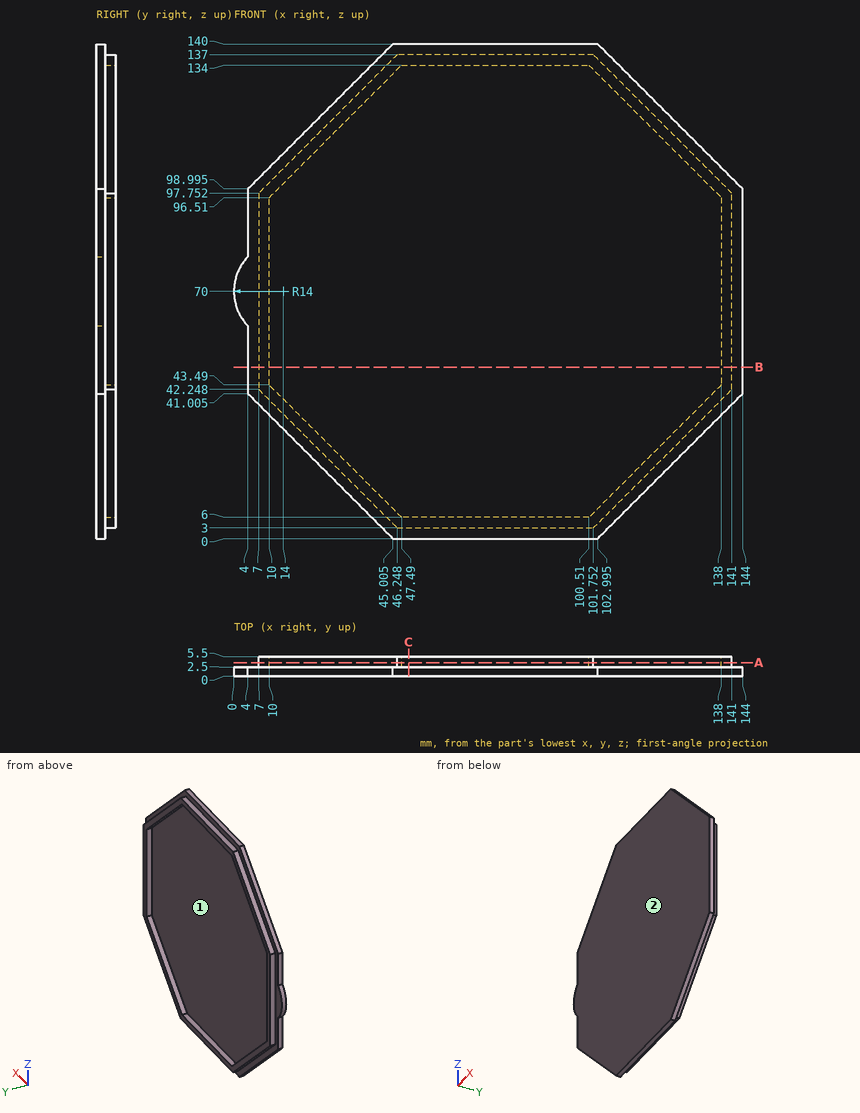
Can you work these out from the drawing? Everything is in mm from the part's minimum corner. Round coordinates to 2 decimals unless told otherwise and drop trailing zeros. Loops run counter-clockwise (first coordinate to the right, second up) from the corner with the lowest first, then second, coordinate; pieces in that order, holes last.
1. If we section it at A-A on y = 3.75: Write out the boundary of the cut face in (x, z), plus the area to 3 significant figures.
Answer list:
outline: (7, 42.25) - (46.25, 3) - (101.75, 3) - (141, 42.25) - (141, 97.75) - (101.75, 137) - (46.25, 137) - (7, 97.75) - close; hole (10, 43.49) - (47.49, 6) - (100.51, 6) - (138, 43.49) - (138, 96.51) - (100.51, 134) - (47.49, 134) - (10, 96.51) - close
area: 1,300 mm2
2. We'd pull the mould along Z, two halves only. Please class the marked faces 1 and 2: +Z half, -Z half, draft (parallel to the pull), parting line (faces both ways), or undercut.
Answer list:
face 1: undercut
face 2: draft
3. For P1, Ø3, axis at x = 79, y = 1.5, coming from the -Z side; P2, Ø2.5, axis at x = 73.5, y = 4, coming from the -Z side; P3, Ø2.5, axis at y = 4, z = 80, coming from the +X side; P4, Ø3, axis at y = 1, z = 92, coming from the -X side, each with a flat end and sliding along its axis, tell me the tip position at first contact or that it passes through.
Answer list:
P1: stops at z = 0
P2: stops at z = 3
P3: stops at x = 141
P4: stops at x = 4
4. If I drill on line 1 along X through (y, z) = (4.3, 64.5); line 2 along Y through (x, z) = (83.5, 60.5); line 3 along Z through (x, y) = (43.5, 2.7), over which ranges is the centre line in solid material (lowest first)?
Answer list:
line 1: x = 7 to 10, 138 to 141
line 2: y = 0 to 2.5
line 3: z = 5.75 to 9.99, 130.01 to 134.25
5. If we section it at C-C on x = 49.5: Write out the boundary of the cut face in (y, z).
Answer list:
outline: (0, 0) - (2.5, 0) - (2.5, 3) - (5.5, 3) - (5.5, 6) - (2.5, 6) - (2.5, 134) - (5.5, 134) - (5.5, 137) - (2.5, 137) - (2.5, 140) - (0, 140) - close
6. If we section it at B-B on z = 48.5: Write out the boundary of the cut face in (x, y).
Answer list:
outline: (4, 0) - (144, 0) - (144, 2.5) - (141, 2.5) - (141, 5.5) - (138, 5.5) - (138, 2.5) - (10, 2.5) - (10, 5.5) - (7, 5.5) - (7, 2.5) - (4, 2.5) - close
